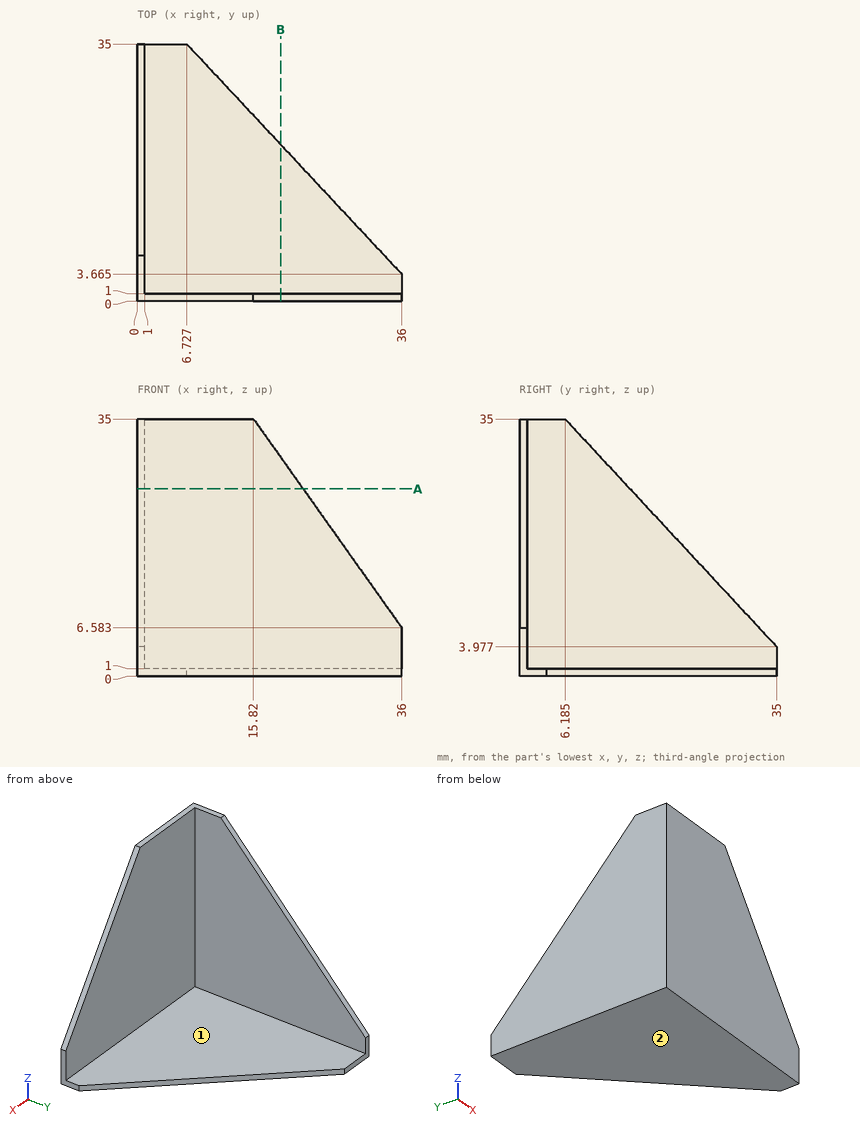
Geometry: see drawing. Coordinates: mm, zero at the bounding-box minimum. A direction names the side the tool comes from. Round coordinates to 2 decimals unless told otherwise and drop trailing zeros. Order: outer loops, then holes, each group sorted by start corner. A loop starts at its lowest first (then second) coordinate and runs counter-clockwise, first axis right, second up. Notation, with made-up numbers: (58, 59) - (84, 59) arc R23 cw to (84, 93) - close; hole circle Ø8 at (44, 43). An arc over 180 degrees is marked (long way). One line per question, with ' | ' between items. Start each with the question number.
1) Set-up query: the marked faces 1 and 2. Return all of +Z, -Z, +X, -X, +Y, -Y with unobstructed straight access to the full face (end or side cutting, diameter ignored); none if empty.
2) Cut plane A-A, the plane z = 25.5. Return the cut outline in (x, y).
3) Cut plane B-B, the plane x = 19.5. Return the cut outline in (y, z).
4) Contact query for flat-ended pins moving along their axis: P1, Ø6, axis at x = 12.5, z = 30.5, coming from the +Y side; P2, Ø12, axis at y = 9.5, z = 25.5, coming from the +X side. Output: stop coordinate, or through.
5) Ray query, probe 1 along X at (y, z) = (11.5, 2.5). Return the intervals inside material, ascending.
Worked out:
1) face 1: +Z, +X, +Y | face 2: -Z, +X, -X, +Y, -Y
2) outline: (0, 0) - (22.57, 0) - (22.57, 1) - (1, 1) - (1, 15.01) - (0, 15.01) - close
3) outline: (0, 0) - (21.33, 0) - (21.33, 1) - (1, 1) - (1, 29.82) - (0, 29.82) - close
4) P1: stops at y = 1 | P2: stops at x = 1
5) probe 1: x = 0 to 1
